For this review, take the finished solid that the model builds, in its own axes (mm). Face numbers are marked on the shaded views. Round coordinates to 2 decimals unless told otherwise and drop trailing zeros. Loops run counter-clockwise (first coordinate to the right, second up) from the corner with the lowest first, then second, coordinate; pieces in that order, holes last.
1) Take a section at B-B (y = 1.75). State the section outline as (x, z) points (3 decimals), then the cut area to 3 significant figures.
2) Take a section at C-C (x = -34.29). State the section outline as (y, z) points (3 decimals), then the cut area to 3 significant figures.
3) Insertion check: pin 1 (5.5 mm diameter, centred on x = -34.29, z = 15.24, fed in from +Y) (3 decimals); pin 2 (2 mm diameter, centred on x = 34.29, z = 15.24, fed in from +Y). Each pin has a flat end and moves straight along its axis. Give the tip position at first contact, or say it passes through.
4) Mouldability with a two-part tool opening along Z and no side actions: class the marked faces 1, 2 and 3 as pulls with the +Z half, pulls with the -Z half, needs draft (parallel to the pull), parting line crosses it, or undercut.
5) Wall thickness on L1, parallel to X at y = 7.5, z = 0 (3 decimals); L2, parallel to X at y = 6, z = 15.24; L3, parallel to Z at x = 34.29, y = 6.5: over which ranges is each line inside the solid? List them lowest first.
6) Take a section at D-D (x = -17). State the section outline as (y, z) points (3 decimals), then the cut area to 3 significant figures.
7) Take a section at A-A (z = 15.24). State the section outline as (x, y) points (3 decimals), then the cut area to 3 significant figures.
```python
from build123d import *

# Parameters (mm, degrees)
SKETCH1_R                                       = 8.89
SKETCH1_R_2                                     = 14.265
BOSS_EXTRUDE1_DEPTH                             = 9.525
CSK_FOR_M3_FLAT_HEAD_MACHINE_SCREW1_D           = 3.4
CSK_FOR_M3_FLAT_HEAD_MACHINE_SCREW1_DEPTH       = 9.99998
CSK_FOR_M3_FLAT_HEAD_MACHINE_SCREW1_CSINK_D     = 6.3
CSK_FOR_M3_FLAT_HEAD_MACHINE_SCREW1_CSINK_ANGLE = 90
CSK_FOR_M3_FLAT_HEAD_MACHINE_SCREW1_TIP         = 1.021463052


with BuildPart() as part:
    # Sketch1 → Boss-Extrude1 (new body)
    with BuildSketch(Plane.XZ):
        with BuildLine():
            Line((-35.56, -19.05), (35.56, -19.05))
            ThreePointArc((35.56, -19.05), (37.356051224, -18.306051224), (38.1, -16.51))
            Line((38.1, -16.51), (38.1, 16.51))
            ThreePointArc((38.1, 16.51), (37.356051224, 18.306051224), (35.56, 19.05))
            Line((35.56, 19.05), (-35.56, 19.05))
            ThreePointArc((-35.56, 19.05), (-37.356051224, 18.306051224), (-38.1, 16.51))
            Line((-38.1, 16.51), (-38.1, -16.51))
            ThreePointArc((-38.1, -16.51), (-37.356051224, -18.306051224), (-35.56, -19.05))
        make_face()
        with Locations(Location((21.59, 0, 0), (0, 0, 270))):
            Circle(SKETCH1_R, mode=Mode.SUBTRACT)
        with Locations(Location((-21.59, 0, 0), (0, 0, 270))):
            Circle(SKETCH1_R_2, mode=Mode.SUBTRACT)
    extrude(amount=-BOSS_EXTRUDE1_DEPTH)

    # CSK for M3 Flat Head Machine Screw1
    with Locations(Plane(origin=(0, 9.525, 0), x_dir=(1, 0, 0), z_dir=(0, 1, 0))):
        with Locations((-34.29, 15.24), (-34.29, -15.24), (34.29, -15.24), (34.29, 15.24)):
            CounterSinkHole(CSK_FOR_M3_FLAT_HEAD_MACHINE_SCREW1_D / 2, CSK_FOR_M3_FLAT_HEAD_MACHINE_SCREW1_CSINK_D / 2, depth=CSK_FOR_M3_FLAT_HEAD_MACHINE_SCREW1_DEPTH, counter_sink_angle=CSK_FOR_M3_FLAT_HEAD_MACHINE_SCREW1_CSINK_ANGLE)
            with Locations((0, 0, -(CSK_FOR_M3_FLAT_HEAD_MACHINE_SCREW1_DEPTH + CSK_FOR_M3_FLAT_HEAD_MACHINE_SCREW1_TIP / 2))):  # 118° drill point
                Cone(0, CSK_FOR_M3_FLAT_HEAD_MACHINE_SCREW1_D / 2, CSK_FOR_M3_FLAT_HEAD_MACHINE_SCREW1_TIP, mode=Mode.SUBTRACT)


solid = part.part
```
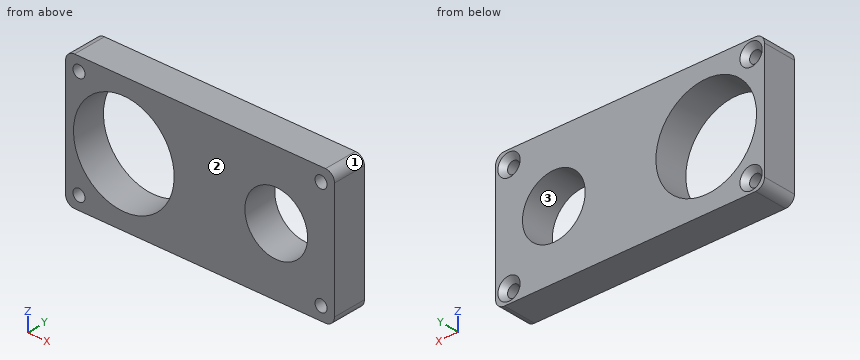
Response:
1. outline: (-38.1, -16.51) arc R2.54 ccw to (-35.56, -19.05) - (35.56, -19.05) arc R2.54 ccw to (38.1, -16.51) - (38.1, 16.51) arc R2.54 ccw to (35.56, 19.05) - (-35.56, 19.05) arc R2.54 ccw to (-38.1, 16.51) - close; hole circle Ø3.4 at (-34.29, -15.24); hole circle Ø3.4 at (-34.29, 15.24); hole circle Ø28.53 at (-21.59, 0); hole circle Ø17.78 at (21.59, 0); hole circle Ø3.4 at (34.29, -15.24); hole circle Ø3.4 at (34.29, 15.24)
1. area: 1,970 mm2
2. outline: (0, -19.05) - (9.525, -19.05) - (9.525, -18.39) - (8.075, -16.94) - (0, -16.94) - close; (0, -13.54) - (8.075, -13.54) - (9.525, -12.09) - (9.525, -6.496) - (0, -6.496) - close; (0, 6.496) - (9.525, 6.496) - (9.525, 12.09) - (8.075, 13.54) - (0, 13.54) - close; (0, 16.94) - (8.075, 16.94) - (9.525, 18.39) - (9.525, 19.05) - (0, 19.05) - close
2. area: 170 mm2
3. pin 1: stops at y = 9.125
3. pin 2: passes through
4. face 1: pulls with the +Z half
4. face 2: needs draft
4. face 3: undercut
5. L1: x = -38.1 to -35.855, -7.325 to 12.7, 30.48 to 38.1
5. L2: x = -38.1 to -35.99, -32.59 to 32.59, 35.99 to 38.1
5. L3: z = -19.05 to -16.94, -13.54 to 13.54, 16.94 to 19.05
6. outline: (0, -19.05) - (9.525, -19.05) - (9.525, -13.506) - (0, -13.506) - close; (0, 13.506) - (9.525, 13.506) - (9.525, 19.05) - (0, 19.05) - close
6. area: 106 mm2
7. outline: (-38.1, 0) - (-35.99, 0) - (-35.99, 8.075) - (-37.44, 9.525) - (-38.1, 9.525) - close; (-32.59, 0) - (32.59, 0) - (32.59, 8.075) - (31.14, 9.525) - (-31.14, 9.525) - (-32.59, 8.075) - close; (35.99, 0) - (38.1, 0) - (38.1, 9.525) - (37.44, 9.525) - (35.99, 8.075) - close
7. area: 657 mm2
